For this review, use the dimensioned drawing (mm, ordinates from the lowest corner) and the shaded views. Round coordinates to 2 decimals unless told otherwise and drop trailing zeros. Order: outer loops, then holes, each group sorted by start corner. A loop starts at its lowest first (then second) coordinate and runs counter-clockwise, first axis right, second up. Notation, with made-up numbers: (51.5, -1.5) -> (59.5, -1.5) arc R18 ccw to (59.5, 29.5) -> close; hole circle Ø9 at (-17.5, 24.5). An arc over 180 degrees is marked (long way). Answer in a Markdown table with one row per item.
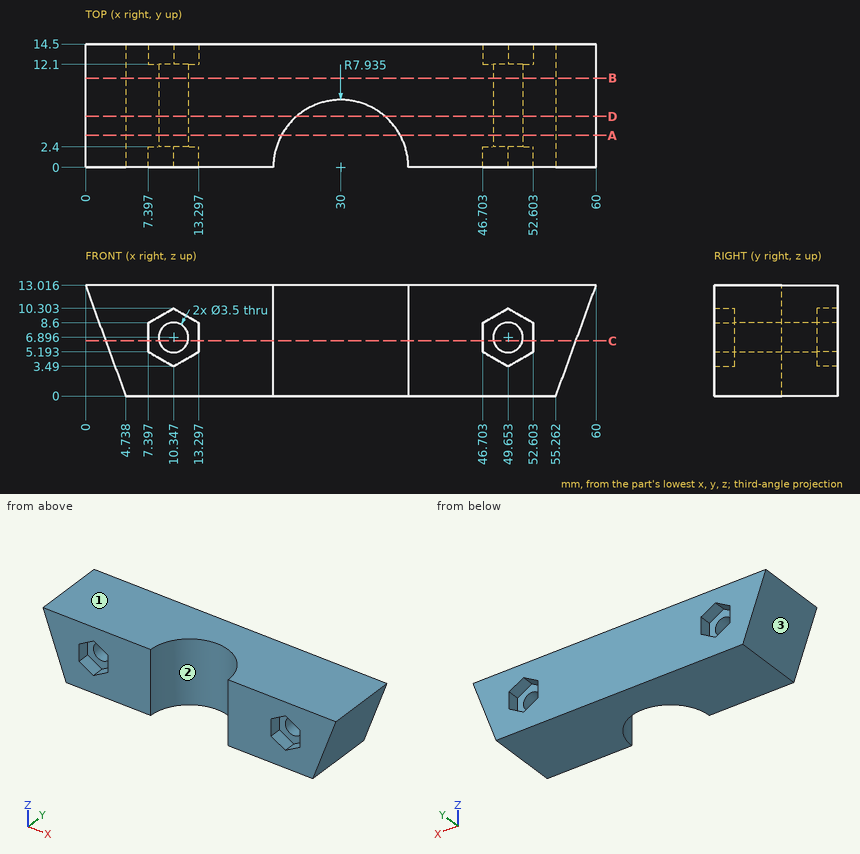
Q1. To check wall thickness, follow probe 1 along X at (y, z) = (1.5, 4) (1 decimal); probe 2 along X at (y, z) = (4.5, 7.25) (1 decimal); probe 3 along X at (y, z) = (11.75, 6.75). State the ranges of each line that lie inside material, in increasing order.
Answer key:
| item | result |
|---|---|
| probe 1 | x = 3.3 to 9.5, 11.2 to 22.2, 37.8 to 48.8, 50.5 to 56.7 |
| probe 2 | x = 2.1 to 8.6, 12.1 to 23.5, 36.5 to 47.9, 51.4 to 57.9 |
| probe 3 | x = 2.28 to 8.6, 12.09 to 47.91, 51.4 to 57.72 |
Q2. The part is to be moulded in two halves that separate along X. For the marked faces 1, 2 and 3, say which applies: +X half, -X half, draft (parallel to the pull), parting line (faces both ways), or undercut.
Answer key:
| item | result |
|---|---|
| face 1 | draft |
| face 2 | undercut |
| face 3 | -X half |
Q3. Take a section at C-C, the plane z = 6.5. Give the number of separate pieces and of enclosed holes in the cut face.
Answer key:
| item | result |
|---|---|
| separate pieces | 3 |
| enclosed holes | 0 |
Q4. Take a section at B-B, the plane y = 10.5. Write out the cut boundary in (x, z), then the cut area to 3 significant figures.
Answer key:
| item | result |
|---|---|
| outline | (0, 13.02) -> (4.74, 0) -> (55.26, 0) -> (60, 13.02) -> close; hole circle Ø3.5 at (10.35, 6.9); hole circle Ø3.5 at (49.65, 6.9) |
| area | 700 mm^2 |
Q5. Take a section at D-D, the plane y = 6. Write out the cut boundary in (x, z).
Answer key:
| item | result |
|---|---|
| outline | (0, 13.02) -> (4.74, 0) -> (24.81, 0) -> (24.81, 13.02) -> close; (35.19, 0) -> (55.26, 0) -> (60, 13.02) -> (35.19, 13.02) -> close; hole circle Ø3.5 at (10.35, 6.9); hole circle Ø3.5 at (49.65, 6.9) |
Q6. Clearance check with flat-ended pins moving along their axes: pin 1 Ø5 at (y, z) = (4, 11.5) entering from -X; pin 2 Ø0.7 at (y, z) = (1, 6.5) entering from -X (1 decimal); pin 3 Ø4 at (x, z) = (10.35, 6.9) entering from -Y; pin 4 Ø3 at (x, z) = (49.65, 6.9) entering from -Y. State where each tip first meets the part, or that it passes through.
Answer key:
| item | result |
|---|---|
| pin 1 | stops at x = 0 |
| pin 2 | stops at x = 2.2 |
| pin 3 | stops at y = 2.4 |
| pin 4 | passes through |
Q7. Take a section at A-A, the plane y = 3.75. Write out the cut boundary in (x, z).
Answer key:
| item | result |
|---|---|
| outline | (0, 13.02) -> (4.74, 0) -> (23.01, 0) -> (23.01, 13.02) -> close; (36.99, 0) -> (55.26, 0) -> (60, 13.02) -> (36.99, 13.02) -> close; hole circle Ø3.5 at (10.35, 6.9); hole circle Ø3.5 at (49.65, 6.9) |
